Autodesk Inventor part; units mm, degrees
ref_plane "YZ Plane" through (0, 0, 0) normal (1, 0, 0) x (0, 1, 0)
ref_plane "XZ Plane" through (0, 0, 0) normal (0, 1, 0) x (-1, 0, 0)
ref_plane "XY Plane" through (0, 0, 0) normal (0, 0, 1) x (1, 0, 0)
sketch "Sketch1" plane through (0, 0, 0) normal (1, 0, 0) x (0, 1, 0)
  line L0 (16, 50) -> (-16, 50)
  line L1 (-16, 50) -> (-16, -42)
  line L2 (-16, -42) -> (16, -42)
  line L3 (16, -42) -> (16, 50)
  circle A0 centre (0, -27) radius 11.75
  line L4 (0, 0) -> (0, -82.2599) construction
  dimension "d0" = 23.5
  dimension "d1" = 27
  dimension "d2" = 50
  dimension "d3" = 32
  dimension "d5" = 42
extrude "Extrusion1" add sketch "Sketch1" along normal blind 4
fillet "Fillet1" radius 3 2 edges at (2, -16, -42) (2, 16, -42)
fillet "Fillet2" radius 6 1 edges at (2, -16, 50)
fillet "Fillet3" radius 6 1 edges at (2, 16, 50)
sketch "Sketch2" plane through (0, 0, 0) normal (-1, 0, 0) x (0, 0, 1)
  line L0 (44, -16) -> (-39, -16)
  line L1 (-39, 16) -> (44, 16)
  line L2 (-1.5, -16) -> (-4.5, -16)
  line L3 (-4.5, -16) -> (-4.5, 16)
  line L4 (-4.5, 16) -> (-1.5, 16)
  line L5 (-1.5, 16) -> (-1.5, -16)
  line L6 (1.5, 16) -> (4.5, 16)
  line L7 (4.5, 16) -> (4.5, -16)
  line L8 (4.5, -16) -> (1.5, -16)
  line L9 (1.5, -16) -> (1.5, 16)
  line L10 (0, -16) -> (0, 16) construction
  point P0 (0, 0)
  point P1 (-1.5, 16)
  point P2 (1.5, 16)
  point P3 (1.5, -16)
  point P4 (4.5, -16)
  dimension "d11" = 3
  dimension "d12" = 3
  dimension "d13" = 3
extrude "Extrusion2" add sketch "Sketch2" along normal blind 15 contours L0 L9 L1 L7 | L0 L3 L1 L5
fillet "Fillet4" radius 3 4 edges at (-15, -16, 3) (-15, -16, -3) (-15, 16, 3) (-15, 16, -3)
sketch "Sketch3" plane through (0, -16, -4.5) normal (0, 0, -1) x (-1, 0, 0)
  circle A0 centre (9, 7) radius 1.75
  circle A1 centre (9, 25) radius 1.75
  line L0 (0, 0) -> (12, 0)
  line L1 (0, 32) -> (12, 32)
  line L2 (15, 29) -> (15, 3)
  circle A2 centre (5, 16) radius 1.75
  point P0 (0, 16)
  dimension "d17" = 3.5
  dimension "d18" = 3.5
  dimension "d19" = 7
  dimension "d20" = 7
  dimension "d21" = 6
  dimension "d22" = 6
  dimension "d23" = 16
  dimension "d24" = 10
  dimension "d25" = 3.5
extrude "Extrusion3" cut sketch "Sketch3" against normal blind 15
properties part number "POUPLY_P5_V2"
The listing builds one solid part. Answer for the finished solid, in the listing's coordinates (mm). A direction names the side the tool comes from. Coordinates: 2 decimals unless noted, no trailing zeros. Write each loop counter-clockwise with the first axis right and the second up, starting at its lowest first coordinate (ties: lowest second). Pieces come first, ordered by that corner, then holes. Notation, with made-up numbers: (19, -34) - (38, -34) arc R5 cw to (38, -30) - close; hole circle Ø6 at (69, -24). An arc over 180 degrees is marked (long way). One line per item, written item: value.
1) Find section C-C (y = 0). Give the vertices of the cut face in (x, z), and give its area (3 significant figures).
Geometry check:
outline: (-15, -4.5) - (-6.75, -4.5) - (-6.75, -1.5) - (-15, -1.5) - close; (-15, 1.5) - (-6.75, 1.5) - (-6.75, 4.5) - (-15, 4.5) - close; (-3.25, -4.5) - (0, -4.5) - (0, -15.25) - (4, -15.25) - (4, 50) - (0, 50) - (0, 4.5) - (-3.25, 4.5) - (-3.25, 1.5) - (0, 1.5) - (0, -1.5) - (-3.25, -1.5) - close; (0, -42) - (4, -42) - (4, -38.75) - (0, -38.75) - close
area: 343 mm2
2) For a pull along Z with two mould halves and no side action, classify faces 3 (the flat face through (0, 0, 0)), 4 (the cylindrical face through (2.028, -14.196, 48.289)), 5 (the flat face through (0, -16, 3)), 6 (the flat face through (-7, 0, -1.5)) as pulls with the +Z half, pulls with the -Z half, needs draft (parallel to the pull), parting line crosses it, or undercut.
Geometry check:
face 3: undercut
face 4: pulls with the +Z half
face 5: needs draft
face 6: undercut
3) Consider line 1 along Y through (x, z) = (-9, 3.6); line 2 along Z through (x, y) = (-9.25, -4); line 3 along X through (y, z) = (-6, 46). Determine where each line is inside the solid, lowest interval first. Write a range as from..to.
Geometry check:
line 1: y = -16..-10.75, -7.25..7.25, 10.75..16
line 2: z = -4.5..-1.5, 1.5..4.5
line 3: x = 0..4
4) Find section B-B (z = -27). Give the vertices of the cut face in (x, y).
Geometry check:
outline: (0, -16) - (4, -16) - (4, -11.75) - (0, -11.75) - close; (0, 11.75) - (4, 11.75) - (4, 16) - (0, 16) - close
5) A tool of negligible diameter and unlimited length cuts with its end or side. For faces 1 (the cylindrical face through (-14.1, 15.14, 3.02)), 2 (the flat face through (-7, 0, -4.5)), from which of +Z, -Z, +X, -X, +Y, -Y can it reach the whole face along a straight path? Write none if from no direction.
Geometry check:
face 1: +Z, -Z, -X, +Y
face 2: -Z, -X, +Y, -Y
6) Each of these flat-tipped pins is pushed along its axis until it touches: pin 1 Ø3 at (x, y) = (-5, 0) entering from -Z; pin 2 Ø7.5 at (x, y) = (-7, -5) entering from -Z; pin 3 Ø9.5 at (y, z) = (3.5, 24) entering from -X; pin 4 Ø2 at (x, y) = (-3.5, -4.5) entering from +Z. Where does it stop, or does it pass through?
Geometry check:
pin 1: passes through
pin 2: stops at z = -4.5
pin 3: stops at x = 0
pin 4: stops at z = 4.5
7) Find section D-D (x = -1.25). Give the vertices of the cut face in (y, z).
Geometry check:
outline: (-16, -4.5) - (16, -4.5) - (16, -1.5) - (-16, -1.5) - close; (-16, 1.5) - (16, 1.5) - (16, 4.5) - (-16, 4.5) - close
8) Find section A-A (x = -5). Give the vertices of the cut face in (y, z), and give its area (3 significant figures).
Geometry check:
outline: (-16, -4.5) - (-1.75, -4.5) - (-1.75, -1.5) - (-16, -1.5) - close; (-16, 1.5) - (-1.75, 1.5) - (-1.75, 4.5) - (-16, 4.5) - close; (1.75, -4.5) - (16, -4.5) - (16, -1.5) - (1.75, -1.5) - close; (1.75, 1.5) - (16, 1.5) - (16, 4.5) - (1.75, 4.5) - close
area: 171 mm2
